from build123d import *

# Parameters (mm, degrees)
SKETCH1_R           = 8.5
SKETCH1_R_2         = 3
BOSS_EXTRUDE1_DEPTH = 6
SKETCH2_W           = 3.5
SKETCH2_H           = 1
SKETCH3_W           = 3.5
SKETCH3_H           = 1


with BuildPart() as part:
    # Sketch1 → Boss-Extrude1 (new body)
    with BuildSketch(Plane.XY):
        Circle(SKETCH1_R)
        Circle(SKETCH1_R_2, mode=Mode.SUBTRACT)
    extrude(amount=BOSS_EXTRUDE1_DEPTH)

    # Sketch2 → Cut-Revolve1 (revolve, cut)
    with BuildSketch(Plane(origin=(0, 0, 0), x_dir=(1, 0, 0), z_dir=(0, 1, 0)), mode=Mode.PRIVATE) as cut_revolve1_sk:
        with Locations((5.75, -0.5)):
            Rectangle(SKETCH2_W, SKETCH2_H)
    revolve(cut_revolve1_sk.sketch.rotate(Axis((0, 0, 0), (0, 0, 1)), 180), axis=Axis((0, 0, 0), (0, 0, 1)), mode=Mode.SUBTRACT)

    # Sketch3 → Cut-Revolve2 (revolve, cut)
    with BuildSketch(Plane(origin=(0, 0, 0), x_dir=(1, 0, 0), z_dir=(0, 1, 0)), mode=Mode.PRIVATE) as cut_revolve2_sk:
        with Locations((5.75, -5.5)):
            Rectangle(SKETCH3_W, SKETCH3_H)
    revolve(cut_revolve2_sk.sketch.rotate(Axis((0, 0, 0), (0, 0, 1)), 180), axis=Axis((0, 0, 0), (0, 0, 1)), mode=Mode.SUBTRACT)


solid = part.part
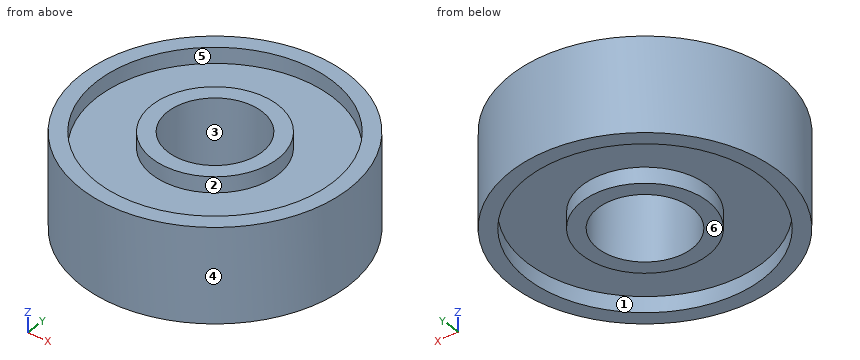
Design review of the part built by this model. Coordinates are the model's own, in mm. Face numbers are marked on the shaded views. A direction names the side the tool comes from. Round coordinates to 2 decimals unless told otherwise and drop trailing zeros. Write each loop counter-clockwise with the first axis right and the second up, starting at its lowest first coordinate (ties: lowest second). Pieces come first, ordered by that corner, then holes. Notation, with made-up numbers: (23.25, 43.25) - (52.25, 43.25) arc R21 cw to (52.25, 77.25) - close; hole circle Ø4 at (38, 39.25). An arc over 180 degrees is marked (long way). Return JSON: item names as keys, results as strings. Group by question number.
Item 1: For probe 1 along Y at (x, z) = (0, 5.55); probe 2 along X at (y, z) = (-0.5, 5.2); probe 3 along Y at (x, z) = (0, 1.8), list the stretches that pass through material, from the lowest coordinate up. Write a range as [from, to].
Item 2: Machinability: for the marked faces 1, 2 and 3, which of the approach directions +Z, -Z, +X, -X, +Y, -Y give a long, thin tool a straight path to every point of the face, cutting with its end or side? Answer none if there is none.
Item 3: We need section A-A on y = 0. Write out the cut boundary in (x, z).
Item 4: We need section D-D on x = 6. Write out the cut boundary in (y, z).
Item 5: The part is to be moulded in two halves that separate along Y. For the marked faces 4, 5 and 6, say which applies: pulls with the +Y half, pulls with the -Y half, needs draft (parallel to the pull), parting line crosses it, or undercut.
Item 6: We need section C-C on z = 0.7. Write out the cut boundary in (x, y), and give its area (3 significant figures).
Model answer:
{
 "1": {"probe 1": "y = [-8.5, -7.5], [-4, -3], [3, 4], [7.5, 8.5]", "probe 2": "x = [-8.49, -7.48], [-3.97, -2.96], [2.96, 3.97], [7.48, 8.49]", "probe 3": "y = [-8.5, -3], [3, 8.5]"},
 "2": {"face 1": "-Z", "face 2": "+Z", "face 3": "+Z, -Z"},
 "3": {"outline": "(-8.5, 0) - (-7.5, 0) - (-7.5, 1) - (-4, 1) - (-4, 0) - (-3, 0) - (-3, 6) - (-4, 6) - (-4, 5) - (-7.5, 5) - (-7.5, 6) - (-8.5, 6) - close; (3, 0) - (4, 0) - (4, 1) - (7.5, 1) - (7.5, 0) - (8.5, 0) - (8.5, 6) - (7.5, 6) - (7.5, 5) - (4, 5) - (4, 6) - (3, 6) - close"},
 "4": {"outline": "(-6.02, 0) - (-4.5, 0) - (-4.5, 1) - (4.5, 1) - (4.5, 0) - (6.02, 0) - (6.02, 6) - (4.5, 6) - (4.5, 5) - (-4.5, 5) - (-4.5, 6) - (-6.02, 6) - close"},
 "5": {"face 4": "parting line crosses it", "face 5": "undercut", "face 6": "needs draft"},
 "6": {"outline": "circle Ø17 at (0, 0); circle Ø8 at (0, 0); hole circle Ø15 at (0, 0); hole circle Ø6 at (0, 0)", "area": "72.3 mm²"}
}
